Geometry: final body of the model. Coordinates: model frame, mm. A direction names the side the tool comes from. Give positions to 0.01 mm unless a question says otherwise; leave off trailing zeros. Order: outer loops, then holes, each group sorted by start corner. A loop starts at its lowest first (then second) coordinate and runs counter-clockwise, first axis right, second up. Notation, with made-up numbers: (56.25, 11.5) - (114.25, 11.5) arc R24 cw to (114.25, 41.5) - close; hole circle Ø4 at (29, 7.5). An arc over 180 degrees is marked (long way). Use one line per item in the form item = value.
from build123d import *

# Parameters (mm, degrees)
F0_W     = 20
F0_H     = 59.5
F0_R     = 2.25
F1_DEPTH = 9.5
F2_W     = 7.5
F2_H     = 3.5
F3_DEPTH = 10
F4_W     = 7.5
F4_H     = 3.5
F5_DEPTH = 10
F6_W     = 20
F6_H     = 79.5
F7_DEPTH = 5
F8_R     = 2.65
F9_DEPTH = 25


with BuildPart() as f1:
    # F0 (on Top) → F1 (new body)
    with BuildSketch(Plane.XY):
        with Locations((-10, -1.060811)):
            Rectangle(F0_W, F0_H)
        with Locations((-10, -26.310811)):
            Circle(F0_R, mode=Mode.SUBTRACT)
        with Locations((-10, 24.189189)):
            Circle(F0_R, mode=Mode.SUBTRACT)
    extrude(amount=F1_DEPTH)

    # F2 (on face) → F3 (cut)
    with BuildSketch(Plane(origin=(0, 28.689189, 0), x_dir=(-1, 0, 0), z_dir=(0, 1, 0))):
        with Locations((10, 4.75)):
            Rectangle(F2_W, F2_H)
    extrude(amount=-F3_DEPTH, mode=Mode.SUBTRACT)

    # F4 (on face) → F5 (cut)
    with BuildSketch(Plane.XZ.offset(30.810811)):
        with Locations((-10, 4.75)):
            Rectangle(F4_W, F4_H)
    extrude(amount=-F5_DEPTH, mode=Mode.SUBTRACT)

    # F6 (on face) → F7 (join)
    with BuildSketch(Plane(origin=(0, 0, 0), x_dir=(1, 0, 0), z_dir=(0, 0, -1))):
        with Locations((-10, 1.060811)):
            Rectangle(F6_W, F6_H)
    extrude(amount=F7_DEPTH)

    # F8 (on face) → F9 (cut)
    with BuildSketch(Plane.XY):
        with Locations((-10, 33.689189)):
            Circle(F8_R)
        with Locations((-10, -35.810811)):
            Circle(F8_R)
    extrude(amount=-F9_DEPTH, mode=Mode.SUBTRACT)


solid = f1.part
(1) Cut plane D-D on y = 25.5. Output: boundary loops of the cut face in (x, z), plus the area to 3 significant figures.
Computed values:
outline = (-20, -5) - (0, -5) - (0, 9.5) - (-8.17, 9.5) - (-8.17, 6.5) - (-6.25, 6.5) - (-6.25, 3) - (-8.17, 3) - (-8.17, 0) - (-11.83, 0) - (-11.83, 3) - (-13.75, 3) - (-13.75, 6.5) - (-11.83, 6.5) - (-11.83, 9.5) - (-20, 9.5) - close
area = 242 mm²
(2) Contact query for flat-ended pins moving along their axis: pin 1 Ø3 at (x, z) = (-11, 5.5) entering from +Y; pin 2 Ø1.5 at (x, z) = (-15.5, 6) entering from -Y; pin 3 Ø1.8 at (x, z) = (-10, 5) entering from -Y. Output: stop coordinate, or through.
Computed values:
pin_1 = 28.69
pin_2 = -30.81
pin_3 = -20.81
(3) Pull-direction query (X, two-part tool) for faces 5 (the face through (-10.29, 26.42, 1.48)), 6 (the face through (-20, -1, 2)), 7 (the face through (-8, -38, 0)); classes: released by +X, released by -X, zero draft, split by the parting line, or undercut.
Computed values:
face_5 = undercut
face_6 = released by -X
face_7 = zero draft
(4) Ray query, line 1 along Y through (x, z) = (-10, 8.1); line 2 along Y through (x, z) = (-10, -2.4); line 3 along X through (y, z) = (24.5, 4.5). Return the intervals inside material, ascending.
Computed values:
line_1 = -30.81 to -28.56, -24.06 to 21.94, 26.44 to 28.69
line_2 = -40.81 to -38.46, -33.16 to 31.04, 36.34 to 38.69
line_3 = -20 to -13.75, -6.25 to 0
(5) Cut plane B-B on z = 5.25. Output: boundary loops of the cut face in (x, y).
Computed values:
outline = (-20, -30.81) - (-13.75, -30.81) - (-13.75, -20.81) - (-6.25, -20.81) - (-6.25, -30.81) - (0, -30.81) - (0, 28.69) - (-6.25, 28.69) - (-6.25, 18.69) - (-13.75, 18.69) - (-13.75, 28.69) - (-20, 28.69) - close
(6) Cut plane A-A on x = -17. Output: boundary loops of the cut face in (y, z).
Computed values:
outline = (-40.81, -5) - (38.69, -5) - (38.69, 0) - (28.69, 0) - (28.69, 9.5) - (-30.81, 9.5) - (-30.81, 0) - (-40.81, 0) - close
(7) Cut plane C-C on x = -10. Give the number of separate pieces and of enclosed holes in the cut face, plus the area to 3 significant figures.
Computed values:
separate_pieces = 5
enclosed_holes = 0
area = 786 mm²
(8) Reachability of faces 1 (the face through (-10.29, -24.08, 7.98)), 2 (the face through (-10, -20.811, 5)), 3 (the face through (-13.75, 24, 5)), 4 (the face through (-8, 36, 0)) from +Z, -Z, +X, -X, +Y, -Y: full face, straight path, thin tool, end or side. Return the list, or none.
Computed values:
face_1 = +Z
face_2 = -Y
face_3 = +Y
face_4 = +Z, +X, -X, +Y
